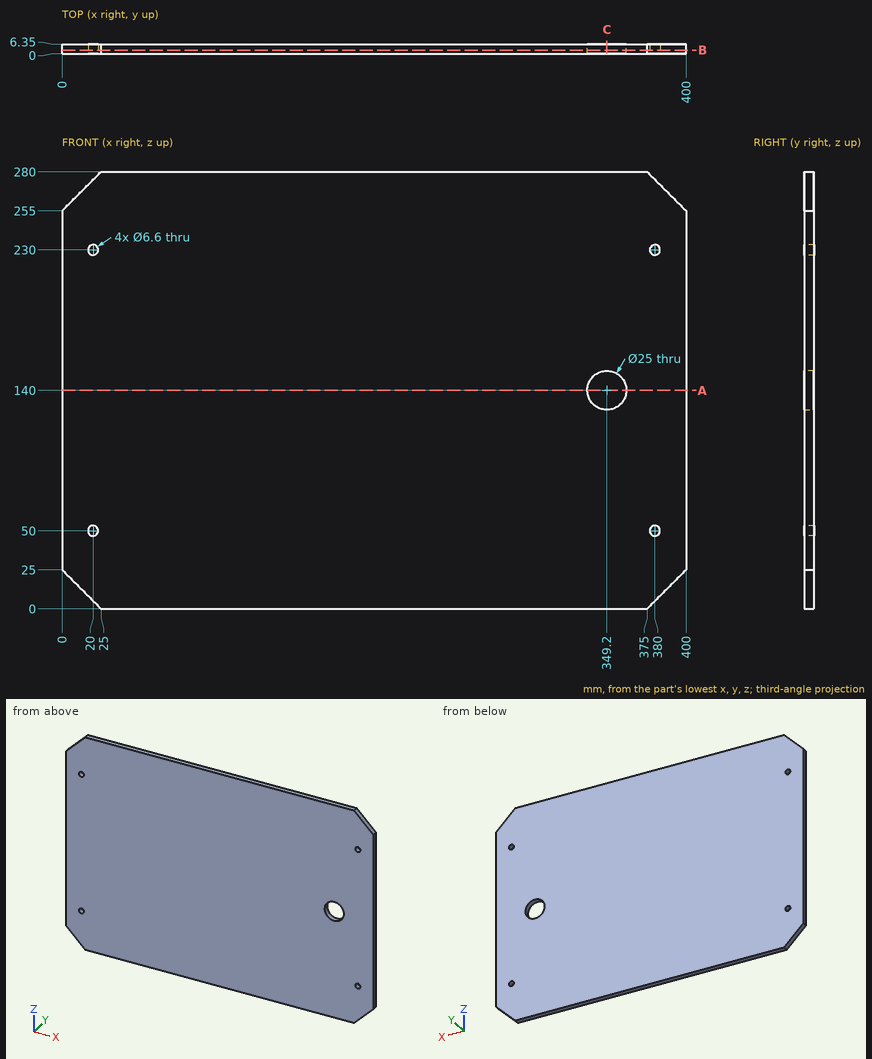
Could you check a few things on this drawing? It's one solid part, dimensions in mm from its lowest x, y, z. Give positions to 0.01 mm unless a question says otherwise; leave off trailing zeros. Order: outer loops, then holes, each group sorted by start corner. A loop starts at its lowest first (then second) coordinate and runs counter-clockwise, first axis right, second up. Notation, with made-up numbers: (-7, 69.25) -> (39, 69.25) arc R37 ccw to (39, 106.25) -> close; hole circle Ø3 at (-16, -36.75). An arc over 180 degrees is marked (long way). Use CSV: the item, a comma, the result in double quotes. Start each with the question number.
Item 1: If I drill on probe 1 along X at (y, z) = (3, 230); probe 2 along Z at (x, y) = (20, 5), over which ranges is the centre line in solid material (lowest first)? Write a range as [from, to].
Item 2: I'm going to push flat-ended pins straight in: P1, Ø6, axis at x = 380, z = 230, coming from the -Y side; P2, Ø10, axis at x = 349, z = 46, coming from the -Y side. Where does each tip first touch, or does it pass through?
Item 3: Suppose I cut it at A-A (z = 140). List the corners of the cut face in (x, y) for me.
Item 4: Suppose I cut it at B-B (y = 2.5). List the corners of the cut face in (x, z) for me, and give its area (3 significant figures).
Item 5: Suppose I cut it at C-C (x = 349.2). List the corners of the cut face in (y, z) for me.
Answer block:
1,probe 1,"x = [0, 16.7], [23.3, 376.7], [383.3, 400]"
1,probe 2,"z = [5, 46.7], [53.3, 226.7], [233.3, 275]"
2,P1,"passes through"
2,P2,"stops at y = 0"
3,outline,"(0, 0) -> (336.7, 0) -> (336.7, 6.35) -> (0, 6.35) -> close; (361.7, 0) -> (400, 0) -> (400, 6.35) -> (361.7, 6.35) -> close"
4,outline,"(0, 25) -> (25, 0) -> (375, 0) -> (400, 25) -> (400, 255) -> (375, 280) -> (25, 280) -> (0, 255) -> close; hole circle Ø6.6 at (20, 50); hole circle Ø6.6 at (20, 230); hole circle Ø25 at (349.2, 140); hole circle Ø6.6 at (380, 50); hole circle Ø6.6 at (380, 230)"
4,area,"110,000 mm^2"
5,outline,"(0, 0) -> (6.35, 0) -> (6.35, 127.5) -> (0, 127.5) -> close; (0, 152.5) -> (6.35, 152.5) -> (6.35, 280) -> (0, 280) -> close"
